For this review, take the finished solid that the model builds, in its own axes (mm). Face numbers are marked on the shaded views. A direction names the side the tool comes from. Coordinates: 2 decimals unless noted, no trailing zeros. Loops run counter-clockwise (first coordinate to the right, second up) from the corner with the lowest first, then second, coordinate; pieces in that order, holes last. Notation, with made-up numbers: M -9.5,-14.5 L 21.5,-14.5 A19 ccw 21.5,22.5 Z; hole C 83.25,42.25 d6. An arc over 180 degrees is marked long. Answer as a JSON object with one key per item and string values. Group by question number.
Item 1: Add section A-A (z = 8). State the section outline as (x, y) points, then the cut area to 3 significant figures.
Item 2: Add section D-D (x = -105). State the section outline as (y, z) points, then the cut area to 3 significant figures.
Item 3: Add section B-B (y = 0). State the section outline as (x, z) points.
Item 4: Add section C-C (z = 0). State the section outline as (x, y) points, then the cut area to 3 significant figures.
Item 5: Insertion check: pin 1 (5 mm diameter, centred on x = -104.5, y = -9.5, fed in from +Z); pin 2 (6 mm diameter, centred on x = -51, y = -7, fed in from +Z); pin 3 (1 mm diameter, centred on x = -51, y = 4, fed in from -Z). Each pin has a flat end and moves straight along its axis. Give the tip position at first contact, or say it passes through.
Item 6: Wall thickness on L1, parallel to X at y = -6, z = -5.5; L2, parallel to X at y = -9.5, z = -1.5; L3, parallel to X at y = 9.5, z = 5.5: over which ranges is each line inside the solid? List them lowest first. Write a range as from..to.
Item 7: Tool access review of the marked faces 1, 2 and 3: name each direction out of +Z, -Z, +X, -X, +Y, -Y from which nothing blocks a thin tool from reaching the whole face with its end or side.
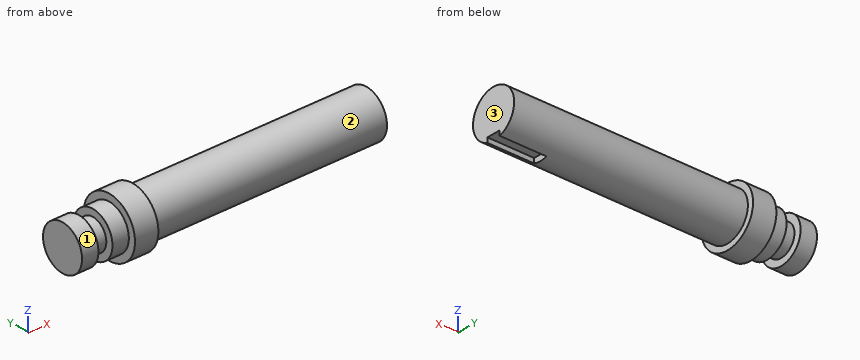
from build123d import *

# Parameters (mm, degrees)
IZIM2_W               = 20
IZIM2_H               = 6
KES_EKSTR_ZYON2_DEPTH = 2.5


with BuildPart() as part:
    # Çizim1 → Döndür1 (revolve)
    with BuildSketch(Plane.XY):
        Polygon((-100, 10), (-100, 12.5), (-110, 12.5), (-110, 9.5), (-117, 9.5), (-117, 6.5), (-123, 6.5), (-123, 9.5), (-130, 9.5), (-130, 0), (0, 0), (0, 10), align=None)
    revolve(axis=Axis((0, 0, 0), (-1, 0, 0)))

    # Çizim2 → Kes-Ekstrüzyon2 (cut)
    with BuildSketch(Plane.XY.offset(-10)):
        with Locations((-10, 0)):
            Rectangle(IZIM2_W, IZIM2_H)
    extrude(amount=KES_EKSTR_ZYON2_DEPTH, mode=Mode.SUBTRACT)


solid = part.part
From the geometry:
{
 "1": {"outline": "M -130,-5.12 L -123,-5.12 L -123,5.12 L -130,5.12 Z; M -117,-5.12 L -110,-5.12 L -110,-9.6 L -100,-9.6 L -100,-6 L 0,-6 L 0,6 L -100,6 L -100,9.6 L -110,9.6 L -110,5.12 L -117,5.12 Z", "area": "1,540 mm²"},
 "2": {"outline": "C 0,0 d25", "area": "491 mm²"},
 "3": {"outline": "M -130,-9.5 L -123,-9.5 L -123,-6.5 L -117,-6.5 L -117,-9.5 L -110,-9.5 L -110,-12.5 L -100,-12.5 L -100,-10 L -20,-10 L -20,-7.5 L 0,-7.5 L 0,10 L -100,10 L -100,12.5 L -110,12.5 L -110,9.5 L -117,9.5 L -117,6.5 L -123,6.5 L -123,9.5 L -130,9.5 Z"},
 "4": {"outline": "M -130,-9.5 L -123,-9.5 L -123,-6.5 L -117,-6.5 L -117,-9.5 L -110,-9.5 L -110,-12.5 L -100,-12.5 L -100,-10 L 0,-10 L 0,10 L -100,10 L -100,12.5 L -110,12.5 L -110,9.5 L -117,9.5 L -117,6.5 L -123,6.5 L -123,9.5 L -130,9.5 Z", "area": "2,590 mm²"},
 "5": {"pin 1": "stops at z = 10.36", "pin 2": "stops at z = 9.17", "pin 3": "stops at z = -9.37"},
 "6": {"L1": "x = -130..-123, -117..0", "L2": "x = -110..0", "L3": "x = -110..-100"},
 "7": {"face 1": "-X", "face 2": "+X", "face 3": "+Z, -Z, +X, +Y, -Y"}
}
